from build123d import *

# Parameters (mm, degrees)
SKETCH_2_W      = 120
SKETCH_2_H      = 200
EXTRUDE_1_DEPTH = 20
EXTRUDE_START   = -7.5
SKETCH_3_R      = 5
EXTRUDE_2_DEPTH = 10
EXTRUDE_START_2 = 5
SKETCH_4_W      = 25
SKETCH_4_H      = 30
SKETCH_4_R      = 5
EXTRUDE_3_DEPTH = 10
EXTRUDE_START_3 = -45
SKETCH_4_2_W    = 25
SKETCH_4_2_H    = 30
SKETCH_4_2_R    = 5
EXTRUDE_4_DEPTH = 10
FILLET_2_R      = 10
FILLET_3_R      = 10
FILLET_4_R      = 5
SKETCH_5_R      = 10
EXTRUDE_5_DEPTH = 30


with BuildPart() as part:
    # Sketch 2 → Extrude 1 (new body)
    with BuildSketch(Plane(origin=(0, 0, 0), x_dir=(1, 0, 0), z_dir=(0, 1, 0))):
        Rectangle(SKETCH_2_W, SKETCH_2_H)
    extrude(amount=EXTRUDE_1_DEPTH)

    # Sketch 3 → Extrude 2 (add)
    with BuildSketch(Plane(origin=(0, 0, 0), x_dir=(0, 0, -1), z_dir=(1, 0, 0)).offset(EXTRUDE_START)):
        with BuildLine():
            ThreePointArc((92.070196982, -19.828078793), (79.999811504, -28.000749672), (67.929286029, -19.828285561))
            Line((67.929286029, -19.828285561), (59.999006327, 0))
            Line((59.999006327, 0), (100, 0))
            Line((100, 0), (92.070196982, -19.828078793))
        make_face()
        with Locations((79.999700158, -15.000749673)):
            Circle(SKETCH_3_R, mode=Mode.SUBTRACT)
    extrude(amount=-EXTRUDE_2_DEPTH)

    # Sketch 4 → Extrude 3 (add)
    with BuildSketch(Plane(origin=(0, 0, 0), x_dir=(0, 0, -1), z_dir=(1, 0, 0)).offset(EXTRUDE_START_2)):
        with Locations((-87.5, -15)):
            Rectangle(SKETCH_4_W, SKETCH_4_H)
        with Locations((-87.5, -15)):
            Circle(SKETCH_4_R, mode=Mode.SUBTRACT)
    extrude_3 = extrude(amount=EXTRUDE_3_DEPTH)

    # Mirror 1: Extrude 3 across plane
    add(extrude_3.mirror(Plane(origin=(0, 0, 0), x_dir=(0, 0, 1), z_dir=(1, 0, 0))))

    # Sketch 4_2 → Extrude 4 (add)
    with BuildSketch(Plane(origin=(0, 0, 0), x_dir=(0, 0, -1), z_dir=(1, 0, 0)).offset(EXTRUDE_START_3)):
        with Locations((-87.5, -15)):
            Rectangle(SKETCH_4_2_W, SKETCH_4_2_H)
        with Locations((-87.5, -15)):
            Circle(SKETCH_4_2_R, mode=Mode.SUBTRACT)
    extrude(amount=-EXTRUDE_4_DEPTH)

    # Fillet 2
    fillet_2_edges = [part.edges().sort_by_distance(p)[0] for p in [
        (-50, -30, 100),
    ]]
    fillet(fillet_2_edges, radius=FILLET_2_R)

    # Fillet 3
    fillet_3_edges = [part.edges().sort_by_distance(p)[0] for p in [
        (-50, -30, 75),
    ]]
    fillet(fillet_3_edges, radius=FILLET_3_R)

    # Fillet 4
    fillet_4_edges = [part.edges().sort_by_distance(p)[0] for p in [
        (-60, 20, 0),
        (0, 20, 100),
        (60, 20, 0),
        (-60, 0, 0),
        (60, 0, 0),
        (0, 20, -100),
    ]]
    fillet(fillet_4_edges, radius=FILLET_4_R)

    # Sketch 5 → Extrude 5 (add)
    with BuildSketch(Plane(origin=(0, 20, 0), x_dir=(1, 0, 0), z_dir=(0, 1, 0))):
        with BuildLine():
            ThreePointArc((49.388864588, -7.793590617), (41.595273971, 0), (49.388864588, 7.793590617))
            ThreePointArc((49.388864588, 7.793590617), (35.355339059, 35.355339059), (7.793590617, 49.388864588))
            ThreePointArc((7.793590617, 49.388864588), (0, 41.595273971), (-7.793590617, 49.388864588))
            ThreePointArc((-7.793590617, 49.388864588), (-35.355339059, 35.355339059), (-49.388864588, 7.793590617))
            ThreePointArc((-49.388864588, 7.793590617), (-41.595273971, 0), (-49.388864588, -7.793590617))
            ThreePointArc((-49.388864588, -7.793590617), (-35.355339059, -35.355339059), (-7.793590617, -49.388864588))
            ThreePointArc((-7.793590617, -49.388864588), (0, -41.595273971), (7.793590617, -49.388864588))
            ThreePointArc((7.793590617, -49.388864588), (35.355339059, -35.355339059), (49.388864588, -7.793590617))
        make_face()
        with Locations(Location((0, 0, 0), (0, 0, 270))):
            Circle(SKETCH_5_R, mode=Mode.SUBTRACT)
    extrude(amount=EXTRUDE_5_DEPTH)


solid = part.part
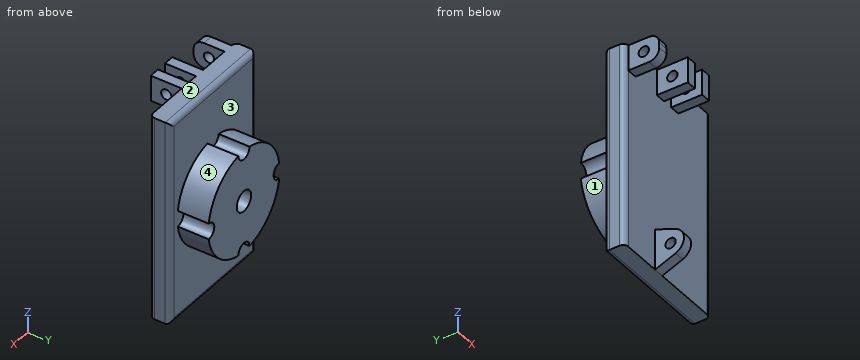
Source: CAD feature listing. Evaluate the final solid. Frame: model axes, mm. Face numbers are marked on the shaded views. A direction names the side the tool comes from. Round coordinates to 2 decimals unless told otherwise and drop trailing zeros. Write each loop counter-clockwise with the first axis right and the second up, starting at its lowest first coordinate (ties: lowest second). Pieces come first, ordered by that corner, then holes. Notation, with made-up numbers: (86, 74.25) - (126, 74.25) arc R11 cw to (126, 92.25) - close; hole circle Ø4 at (2, 49.5). An arc over 180 degrees is marked (long way). Use CSV: the item, a comma, the result in double quotes. Start each with the question number.
(1) First-contact query: pin 1 Ø5 at (x, y) = (-9.5, -8.5) entering from -Z; pin 2 Ø6 at (y, z) = (30, 24) entering from -X; pin 3 Ø5 at (x, z) = (5, 19.5) entering from -Y; pin 4 Ø3 at (y, z) = (4.5, -55) entering from +X. Flat tips, straight axial feed; report the tip coordinate or a pass-through.
(2) Set-up query: the marked faces 1, 2, 3 and 4. Return all of +Z, -Z, +X, -X, +Y, -Y with unobstructed straight access to the full face (end or side cutting, diameter ignored); none if empty.
(3) Cut plane D-D, the plane z = 64. Return loops of the section in (x, y).
(4) Material intervals for probe 1 along Y at (x, z) = (13.25, 87.5); probe 2 along Y at (x, z) = (-28.5, -64); probe 3 along X at (y, z) = (41, 0), sorted ascending. Write a range as [from, to].
(5) Cut plane C-C, the plane y = -23.5. Return loops of the section in (x, z), and give its area (3 significant figures).
(6) Cut plane A-A, the plane z = 87.5. Give the number of separate pieces and of enclosed holes in the cut face, and give its area (3 significant figures).
Geometry says:
1,pin 1,"z = -97.6"
1,pin 2,"x = -45.38"
1,pin 3,"y = 0"
1,pin 4,"x = 60"
2,face 1,"-Z, -X, +Y"
2,face 2,"+Z, +X, -X, +Y, -Y"
2,face 3,"+Y"
2,face 4,"+Z, +X, +Y"
3,outline,"(-60, 5) arc R5 ccw to (-55, 0) - (55, 0) arc R5 ccw to (60, 5) - (60, 15) arc R5 ccw to (55, 20) - (-55, 20) arc R5 ccw to (-60, 15) - close"
4,probe 1,"[-30, -20], [-10, 20]"
4,probe 2,"[0, 20]"
4,probe 3,"[-41.6, -10], [10, 41.6]"
5,outline,"(-55, 75.63) - (-45, 75.63) - (-45, 99.37) - (-55, 99.37) - close; (-17.5, -89.84) - (-7.5, -89.84) - (-7.5, -70.16) - (-17.5, -70.16) - close; (-15, 75) - (-5, 75) - (-5, 100) - (-15, 100) - close; (5, 75) - (15, 75) - (15, 100) - (5, 100) - close"
5,area,"934 mm²"
6,separate pieces,"4"
6,enclosed holes,"0"
6,area,"2,980 mm²"
